Input: dimensioned drawing with shaded views. Units: mm. Origin: part minimum x, y, z. A direction names the side the tool comes from. Coordinates: 2 decimals unless noted, no trailing zeros. Loops run counter-clockwise (first coordinate to the right, second up) from the corner with the lowest first, then second, coordinate; pieces in that order, holes last.
Item 1: Pull-direction query (X, two-part tool) for the marked faces 6, 7 and 8; classes: released by +X, released by -X, zero draft, split by the parting line, or undercut.
Item 2: Section D-D on z = 0.3. Return loops of the section in (x, y), and give its area (3 significant figures).
Item 3: Section B-B on x = 12.5. Return loops of the section in (y, z), and give its area (3 significant figures).
Item 4: Section A-A on y = 6.75. Return loops of the section in (x, z).
Item 5: Contact query for flat-ended pins moving along their axis: P1, Ø1.2, axis at y = 2.5, z = 2.5, coming from the +X side; P2, Ø1.6, axis at x = 4, z = 3.5, coming from the +Y side; P3, Ø1.4, axis at y = 9, z = 3, coming from the +X side. Output: stop coordinate, or through.
Item 6: Ray query, line 1 along X through (y, z) = (4, 4.5); line 2 along Y through (x, z) = (12.75, 2.8); line 3 along X through (y, z) = (10, 0.75). Return the intervals inside material, ascending.
Item 7: Reachability of the marked faces 1, 2, 3, 4 and 5 from +Z, -Z, +X, -X, +Y, -Y: full face, straight path, thin tool, end or side. Return the list, or none.
Item 8: Section C-C on z = 3. Return loops of the section in (x, y).
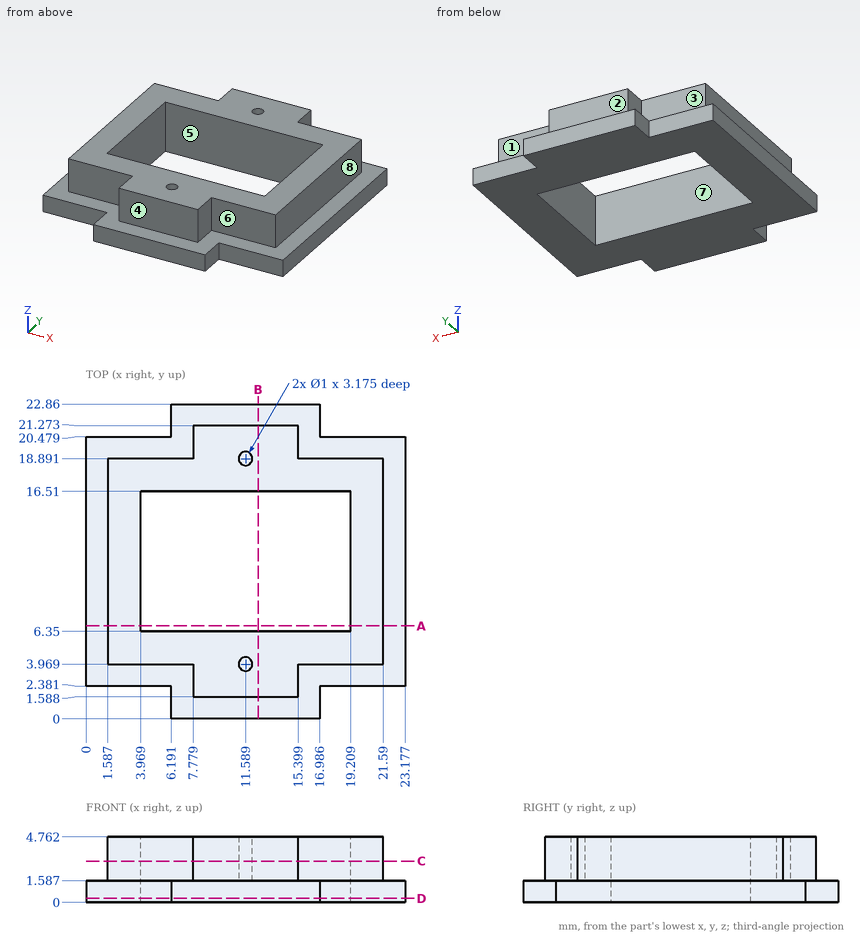
Results found:
1. face 6: zero draft
1. face 7: undercut
1. face 8: released by +X
2. outline: (0, 2.38) - (6.19, 2.38) - (6.19, 0) - (16.99, 0) - (16.99, 2.38) - (23.18, 2.38) - (23.18, 20.48) - (16.99, 20.48) - (16.99, 22.86) - (6.19, 22.86) - (6.19, 20.48) - (0, 20.48) - close; hole (3.97, 6.35) - (19.21, 6.35) - (19.21, 16.51) - (3.97, 16.51) - close
2. area: 316 mm2
3. outline: (0, 0) - (6.35, 0) - (6.35, 4.76) - (1.59, 4.76) - (1.59, 1.59) - (0, 1.59) - close; (16.51, 0) - (22.86, 0) - (22.86, 1.59) - (21.27, 1.59) - (21.27, 4.76) - (16.51, 4.76) - close
3. area: 50.4 mm2
4. outline: (0, 0) - (3.97, 0) - (3.97, 4.76) - (1.59, 4.76) - (1.59, 1.59) - (0, 1.59) - close; (19.21, 0) - (23.18, 0) - (23.18, 1.59) - (21.59, 1.59) - (21.59, 4.76) - (19.21, 4.76) - close
5. P1: stops at x = 15.4
5. P2: stops at y = 18.89
5. P3: stops at x = 21.59
6. line 1: x = 1.59 to 11.09, 12.09 to 21.59
6. line 2: y = 1.59 to 6.35, 16.51 to 21.27
6. line 3: x = 0 to 3.97, 19.21 to 23.18
7. face 1: +Z, +X, +Y
7. face 2: +Z, +X, -X, +Y
7. face 3: +Z, -X, +Y
7. face 4: +Z, +X, -X, -Y
7. face 5: +Z, -Z
8. outline: (1.59, 3.97) - (7.78, 3.97) - (7.78, 1.59) - (15.4, 1.59) - (15.4, 3.97) - (21.59, 3.97) - (21.59, 18.89) - (15.4, 18.89) - (15.4, 21.27) - (7.78, 21.27) - (7.78, 18.89) - (1.59, 18.89) - close; hole (3.97, 6.35) - (19.21, 6.35) - (19.21, 16.51) - (3.97, 16.51) - close; hole circle Ø1 at (11.59, 3.97); hole circle Ø1 at (11.59, 18.89)
